from build123d import *

# Parameters (mm, degrees)
SKETCH1_W                                        = 152.4
SKETCH1_H                                        = 152.4
SKETCH1_R                                        = 3.2639
BOSS_EXTRUDE1_DEPTH                              = 6.35
SKETCH3_R                                        = 6.342
SKETCH4_R                                        = 0.5
SKETCH7_R                                        = 6.342
SKETCH8_R                                        = 0.5
F_8_32_TAPPED_HOLE1_D                            = 3.4544
CBORE_FOR_1_4_SOCKET_HEAD_CAP_SCREW1_D           = 6.5278
CBORE_FOR_1_4_SOCKET_HEAD_CAP_SCREW1_CBORE_D     = 11.1125
CBORE_FOR_1_4_SOCKET_HEAD_CAP_SCREW1_CBORE_DEPTH = 3.175
FILLET1_R                                        = 1


with BuildPart() as part:
    # Sketch1 → Boss-Extrude1 (new body)
    # profile 1 of 13: a face of its own
    with BuildSketch(Plane(origin=(0, 0, 0), x_dir=(1, 0, 0), z_dir=(0, 1, 0))):
        with Locations((76.2, -76.2)):
            Rectangle(SKETCH1_W, SKETCH1_H)
        with Locations((12.7, -38.1)):
            Circle(SKETCH1_R, mode=Mode.SUBTRACT)
        with Locations((12.7, -114.3)):
            Circle(SKETCH1_R, mode=Mode.SUBTRACT)
        with Locations((38.1, -139.7)):
            Circle(SKETCH1_R, mode=Mode.SUBTRACT)
        with Locations((114.3, -139.7)):
            Circle(SKETCH1_R, mode=Mode.SUBTRACT)
        with Locations((139.7, -114.3)):
            Circle(SKETCH1_R, mode=Mode.SUBTRACT)
        with Locations((139.7, -38.1)):
            Circle(SKETCH1_R, mode=Mode.SUBTRACT)
        with Locations((114.3, -12.7)):
            Circle(SKETCH1_R, mode=Mode.SUBTRACT)
        with Locations((38.1, -12.7)):
            Circle(SKETCH1_R, mode=Mode.SUBTRACT)
        with Locations((12.7, -139.7)):
            Circle(SKETCH1_R, mode=Mode.SUBTRACT)
        with Locations((139.7, -139.7)):
            Circle(SKETCH1_R, mode=Mode.SUBTRACT)
        with Locations((139.7, -12.7)):
            Circle(SKETCH1_R, mode=Mode.SUBTRACT)
        with Locations((12.7, -12.7)):
            Circle(SKETCH1_R, mode=Mode.SUBTRACT)
    # profile 2 of 13: a face of its own
    with BuildSketch(Plane(origin=(0, 0, 0), x_dir=(1, 0, 0), z_dir=(0, 1, 0))):
        with Locations((12.7, -12.7)):
            Circle(SKETCH1_R)
    # profile 3 of 13: a face of its own
    with BuildSketch(Plane(origin=(0, 0, 0), x_dir=(1, 0, 0), z_dir=(0, 1, 0))):
        with Locations((139.7, -12.7)):
            Circle(SKETCH1_R)
    # profile 4 of 13: a face of its own
    with BuildSketch(Plane(origin=(0, 0, 0), x_dir=(1, 0, 0), z_dir=(0, 1, 0))):
        with Locations((139.7, -139.7)):
            Circle(SKETCH1_R)
    # profile 5 of 13: a face of its own
    with BuildSketch(Plane(origin=(0, 0, 0), x_dir=(1, 0, 0), z_dir=(0, 1, 0))):
        with Locations((12.7, -139.7)):
            Circle(SKETCH1_R)
    # profile 6 of 13: a face of its own
    with BuildSketch(Plane(origin=(0, 0, 0), x_dir=(1, 0, 0), z_dir=(0, 1, 0))):
        with Locations((38.1, -12.7)):
            Circle(SKETCH1_R)
    # profile 7 of 13: a face of its own
    with BuildSketch(Plane(origin=(0, 0, 0), x_dir=(1, 0, 0), z_dir=(0, 1, 0))):
        with Locations((12.7, -38.1)):
            Circle(SKETCH1_R)
    # profile 8 of 13: a face of its own
    with BuildSketch(Plane(origin=(0, 0, 0), x_dir=(1, 0, 0), z_dir=(0, 1, 0))):
        with Locations((139.7, -38.1)):
            Circle(SKETCH1_R)
    # profile 9 of 13: a face of its own
    with BuildSketch(Plane(origin=(0, 0, 0), x_dir=(1, 0, 0), z_dir=(0, 1, 0))):
        with Locations((114.3, -12.7)):
            Circle(SKETCH1_R)
    # profile 10 of 13: a face of its own
    with BuildSketch(Plane(origin=(0, 0, 0), x_dir=(1, 0, 0), z_dir=(0, 1, 0))):
        with Locations((139.7, -114.3)):
            Circle(SKETCH1_R)
    # profile 11 of 13: a face of its own
    with BuildSketch(Plane(origin=(0, 0, 0), x_dir=(1, 0, 0), z_dir=(0, 1, 0))):
        with Locations((114.3, -139.7)):
            Circle(SKETCH1_R)
    # profile 12 of 13: a face of its own
    with BuildSketch(Plane(origin=(0, 0, 0), x_dir=(1, 0, 0), z_dir=(0, 1, 0))):
        with Locations((12.7, -114.3)):
            Circle(SKETCH1_R)
    # profile 13 of 13: a face of its own
    with BuildSketch(Plane(origin=(0, 0, 0), x_dir=(1, 0, 0), z_dir=(0, 1, 0))):
        with Locations((38.1, -139.7)):
            Circle(SKETCH1_R)
    extrude(amount=BOSS_EXTRUDE1_DEPTH)

    # Sketch3 → Cut-Loft1 section 0
    with BuildSketch(Plane(origin=(0, 6.35, 0), x_dir=(1, 0, 0), z_dir=(0, 1, 0))):
        with Locations((12.7, -12.7)):
            Circle(SKETCH3_R)
    # Sketch4 → Cut-Loft1 section 1
    with BuildSketch(Plane(origin=(0, 0.508, 0), x_dir=(1, 0, 0), z_dir=(0, 1, 0))):
        with Locations((12.7, -12.7)):
            Circle(SKETCH4_R)
    loft(mode=Mode.SUBTRACT)

    # Cut-Loft2: read off the stored shape, not the designer's step
    # Cut-Loft2: loft between two sections, ruled curve by curve
    cut_loft2_from = [
        Edge.make_bspline([(7.199053533, 6.35, 142.856034215), (0.886985103, 6.35, 131.85414128), (11.888878038, 6.35, 125.542072851), (18.200946467, 6.35, 136.543965785), (24.513014897, 6.35, 147.54585872), (13.511121962, 6.35, 153.857927149), (7.199053533, 6.35, 142.856034215)], [0, 0, 0, 0, 0.5, 0.5, 0.5, 1, 1, 1, 1], 3, [1, 0.333333333, 0.333333333, 1, 0.333333333, 0.333333333, 1]),
    ]
    cut_loft2_to = [
        Edge.make_bspline([(12.346224535, 0.508, 140.053331177), (11.639562182, 0.508, 139.345780247), (12.347113112, 0.508, 138.639117893), (13.053775465, 0.508, 139.346668823), (13.760437818, 0.508, 140.054219753), (13.052886888, 0.508, 140.760882107), (12.346224535, 0.508, 140.053331177)], [0, 0, 0, 0, 0.5, 0.5, 0.5, 1, 1, 1, 1], 3, [1, 0.333333333, 0.333333333, 1, 0.333333333, 0.333333333, 1]),
    ]
    cut_loft2 = Solid(Shell([*[Face.make_surface_from_curves(cut_loft2_from[k], cut_loft2_to[k]) for k in range(1)], Face(Wire(cut_loft2_from)), Face(Wire(cut_loft2_to))]))
    add(cut_loft2, mode=Mode.SUBTRACT)

    # Sketch7 → Cut-Loft4 section 0
    with BuildSketch(Plane(origin=(0, 6.35, 0), x_dir=(1, 0, 0), z_dir=(0, 1, 0))):
        with Locations((139.7, -76.2)):
            Circle(SKETCH7_R)
    # Sketch8 → Cut-Loft4 section 1
    with BuildSketch(Plane(origin=(0, 0.508, -1.35), x_dir=(1, 0, 0), z_dir=(0, -1, 0))):
        with Locations((139.7, 77.55)):
            Circle(SKETCH8_R)
    loft(mode=Mode.SUBTRACT)

    # #8-32 Tapped Hole1 (through all)
    with Locations(Plane(origin=(16.7, 0, 76.2), x_dir=(0, 0, -1), z_dir=(0, -1, 0))):
        with Locations((0, 0), (18.3382, 77.8382), (-18.3382, 77.8382)):
            Hole(F_8_32_TAPPED_HOLE1_D / 2)

    # CBORE for 1/4 Socket Head Cap Screw1 (through all)
    with Locations(Plane(origin=(38.1, 6.35, 12.7), x_dir=(0, 0, 1), z_dir=(0, 1, 0))):
        with Locations((0, 0), (25.4, -25.4), (0, 76.2), (25.4, 101.6), (101.6, 101.6), (127, 76.2), (127, 0), (101.6, -25.4)):
            CounterBoreHole(CBORE_FOR_1_4_SOCKET_HEAD_CAP_SCREW1_D / 2, CBORE_FOR_1_4_SOCKET_HEAD_CAP_SCREW1_CBORE_D / 2, CBORE_FOR_1_4_SOCKET_HEAD_CAP_SCREW1_CBORE_DEPTH)

    # Fillet1
    fillet1_edges = [part.edges().sort_by_distance(p)[0] for p in [
        (152.4, 3.175, 152.4),
        (0, 3.175, 152.4),
        (0, 3.175, 0),
        (152.4, 3.175, 0),
    ]]
    fillet(fillet1_edges, radius=FILLET1_R)


solid = part.part
Part model, mm, in its own coordinate system. A direction names the side the tool comes from. Give positions to 0.01 mm unless a question says otherwise; leave off trailing zeros. Order: outer loops, then holes, each group sorted by start corner. A loop starts at its lowest first (then second) coordinate and runs counter-clockwise, first axis right, second up. Notation, with made-up numbers: (-34.5, 59) -> (15.5, 59) arc R20 cw to (15.5, 80) -> close; hole circle Ø6 at (-23.5, 18). An arc over 180 degrees is marked (long way). Use one line per item in the form item = value.
(1) Saw through at A-A (z = 38.1). Write the cut outline in (x, y) (3 decimals).
Solution:
outline = (0, 0) -> (9.436, 0) -> (9.436, 3.175) -> (7.144, 3.175) -> (7.144, 6.35) -> (0, 6.35) -> close; (15.964, 0) -> (136.436, 0) -> (136.436, 3.175) -> (134.144, 3.175) -> (134.144, 6.35) -> (18.256, 6.35) -> (18.256, 3.175) -> (15.964, 3.175) -> close; (142.964, 0) -> (152.4, 0) -> (152.4, 6.35) -> (145.256, 6.35) -> (145.256, 3.175) -> (142.964, 3.175) -> close
(2) Pull direction X, two halves, no side cores. Call faces 1 (the face through (75, 3, 152.4)), 2 (the face through (152.4, 3, 77)), 3 (the face through (141, 1.4, 76.7)): +X half, -X half, draft (parallel to the pull), parting line (faces both ways), or undercut.
Solution:
face_1 = draft
face_2 = +X half
face_3 = undercut
(3) Saw through at B-B (x = 114.3). Write the cut outline in (y, z) (3 decimals).
Solution:
outline = (0, 0) -> (6.35, 0) -> (6.35, 7.144) -> (3.175, 7.144) -> (3.175, 9.436) -> (0, 9.436) -> close; (0, 15.964) -> (3.175, 15.964) -> (3.175, 18.256) -> (6.35, 18.256) -> (6.35, 134.144) -> (3.175, 134.144) -> (3.175, 136.436) -> (0, 136.436) -> close; (0, 142.964) -> (3.175, 142.964) -> (3.175, 145.256) -> (6.35, 145.256) -> (6.35, 152.4) -> (0, 152.4) -> close
(4) Flat gauge pin, fed straight in: P1, Ø0.8, axis at x = 12.5, z = 140, coming from the +Y side. Where does the tip first touch, or does it go through?
Solution:
P1 = 0.77
(5) Tool access for faces 4 (the face through (39.77, 4.78, 145)), 5 (the face through (40.852, 1.565, 137.945)): list every direction of +Z, -Z, +X, -X, +Y, -Y with a clear straight run to the whole face (end or side of a thin tool).
Solution:
face_4 = +Y
face_5 = +Y, -Y
(6) Drill centre lines: line 1 (X direction, y = 1.4, z = 38.1); line 2 (X direction, y = 4.35, z = 38.1); line 3 (X direction, y = 1.6, z = 139.7). Where is each one in solid material? Low to high. Write a range as from..to.
Solution:
line_1 = 0..9.44, 15.96..136.44, 142.96..152.4
line_2 = 0..7.14, 18.26..134.14, 145.26..152.4
line_3 = 0..11.12, 14.28..34.84, 41.36..111.04, 117.56..152.4
(7) Saw through at C-C (y = 4.5). Count the separate pieces of the cut face and the enclosed holes in it, then the cut area to 3 significant figures.
Solution:
separate_pieces = 1
enclosed_holes = 14
area = 22,200 mm²
